The figure shows three views and two pictorial views of one solid part (mm, origin at its lowest corner). Answer the questions. A direction names the side the tool comes from. Round coordinates to 2 decimals unless told otherwise and drop trailing zeros. Order: outer loops, then holes, each group sorted by start corner. A loop starts at its lowest first (then second) coordinate and runs counter-clockwise, first axis right, second up. Notation, with made-up numbers: (11, 79) - (27, 79) arc R21 ccw to (27, 90) - close; hole circle Ø7 at (54, 80.25). An arc over 180 degrees is marked (long way). Answer as a JSON object with one key per item and string values. Group by question number.
Q1. A cutting plane is placed at D-D on x = 6.75. Determine the outline of the cut face in (y, z).
Q2. A tool of negligible diameter and unlimited length cuts with its end or side. For the marked faces 1, 2 and 3, from which of +Z, -Z, +X, -X, +Y, -Y can it reach the whole face along a straight path? Write none if from no direction.
Q3. The mould has two halves that part along Y. Classify the marked faces 4, 5 and 6: pulls with the +Y half, pulls with the -Y half, needs draft (parallel to the pull), parting line crosses it, or undercut.
Q4. Consider line 1 (Y direction, x = 10, z = 0.8); line 2 (Y direction, x = 13.5, z = 2.5); line 3 (X direction, y = 4, z = 2.6). Determine where each line is inside the solid, lowest interval first.
Q5. A cutting plane is placed at A-A on x = 3.75. Determine the outline of the cut face in (y, z).
Q6. Given pin 1 Ø0.6 at (y, z) = (11, 1.5) entering from +X; pin 2 Ø1 at (x, z) = (5, 2.5) entering from +Y; pin 3 Ø1 at (y, z) = (17, 0.5) entering from -X; pin 4 Ø4 at (x, y) = (3, 5) entering from -Z, each flat-ended and moving along its own axis, determine where each tip first touches the part or whether it passes through.
Q7. A cutting plane is placed at C-C on y = 10. Determine the outline of the cut face in (x, z), and give its area (3 significant figures).
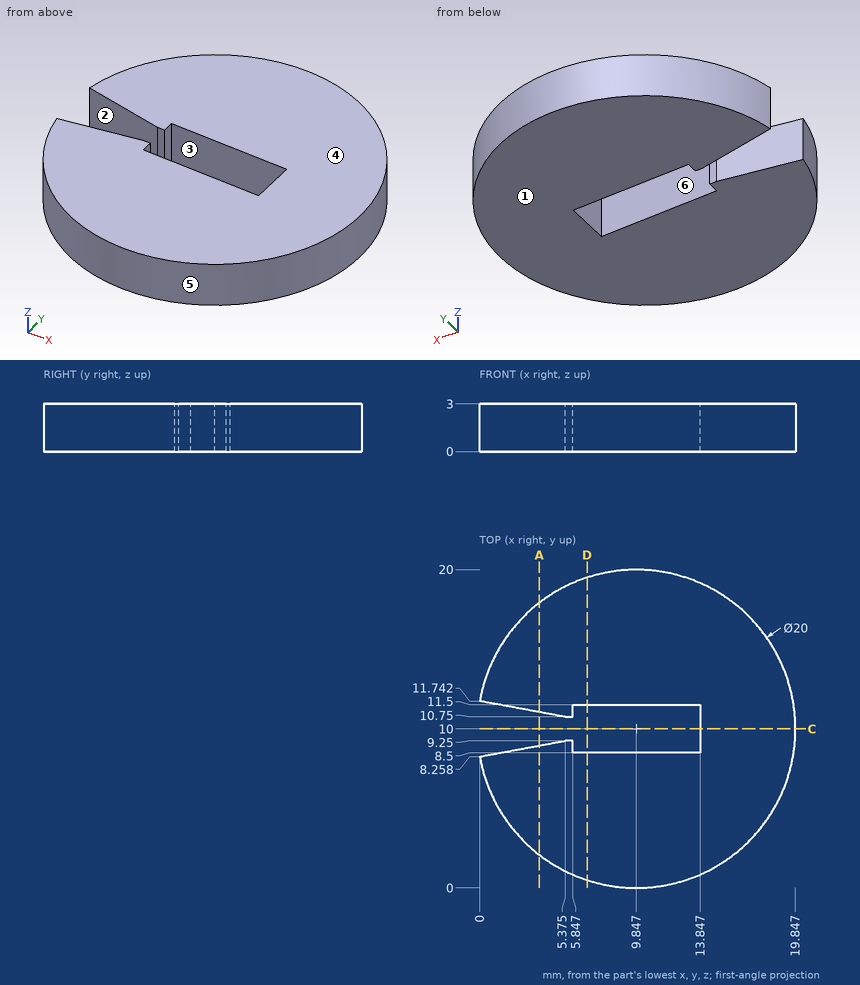
Result set:
{
 "1": {"outline": "(0.49, 0) - (8.5, 0) - (8.5, 3) - (0.49, 3) - close; (11.5, 0) - (19.51, 0) - (19.51, 3) - (11.5, 3) - close"},
 "2": {"face 1": "-Z, +X, -X, +Y, -Y", "face 2": "+Z, -Z, -X", "face 3": "+Z, -Z"},
 "3": {"face 4": "needs draft", "face 5": "parting line crosses it", "face 6": "undercut"},
 "4": {"line 1": "y = 0 to 8.5, 11.5 to 20", "line 2": "y = 0.69 to 8.5, 11.5 to 19.31", "line 3": "x = 1.85 to 17.85"},
 "5": {"outline": "(2.07, 0) - (8.95, 0) - (8.95, 3) - (2.07, 3) - close; (11.05, 0) - (17.93, 0) - (17.93, 3) - (11.05, 3) - close"},
 "6": {"pin 1": "stops at x = 19.82", "pin 2": "stops at y = 19.01", "pin 3": "stops at x = 2.25", "pin 4": "stops at z = 0"},
 "7": {"outline": "(13.85, 0) - (19.85, 0) - (19.85, 3) - (13.85, 3) - close", "area": "18.0 mm²"}
}
